```python
from build123d import *

# Parameters (mm, degrees)
F1_DEPTH      = 54.102
F1_DEPTH_BACK = 31.75
F3_DEPTH      = 66.802
F4_R          = 6.35
F6_D          = 25.4
F8_D          = 12.7


with BuildPart() as f1:
    # F0 (on Right) → F1 (new body, two sides)
    with BuildSketch(Plane.YZ) as f1_sk:
        with BuildLine():
            Line((-209.55, 0), (0, 0))
            Line((0, 0), (0, 66.802))
            Line((0, 66.802), (-12.7, 66.802))
            Line((-12.7, 66.802), (-12.7, 16.002))
            Line((-12.7, 16.002), (-69.85, 16.002))
            Line((-69.85, 16.002), (-69.85, 60.452))
            Line((-69.85, 60.452), (-82.55, 60.452))
            Line((-82.55, 60.452), (-82.55, 24.892))
            ThreePointArc((-82.55, 24.892), (-85.153821, 18.605821), (-91.44, 16.002))
            Line((-91.44, 16.002), (-209.55, 16.002))
            Line((-209.55, 16.002), (-209.55, 0))
        make_face()
    extrude(amount=F1_DEPTH)
    extrude(f1_sk.sketch, amount=-F1_DEPTH_BACK)

    # F2 (on Top) → F3 (cut)
    with BuildSketch(Plane.XY):
        with BuildLine():
            Line((31.75, -209.55), (54.102, -209.55))
            Line((54.102, -209.55), (54.102, -12.7))
            Line((54.102, -12.7), (44.45, -12.7))
            ThreePointArc((44.45, -12.7), (35.469744, -16.419744), (31.75, -25.4))
            Line((31.75, -25.4), (31.75, -209.55))
        make_face()
    extrude(amount=F3_DEPTH, mode=Mode.SUBTRACT)

    # F4
    f4_edges = [f1.edges().sort_by_distance(p)[0] for p in [
        (54.102, -6.35, 0),
        (54.102, -6.35, 66.802),
    ]]
    fillet(f4_edges, radius=F4_R)

    # F6 (through all)
    with Locations(Plane.XY.offset(16.002)):
        with Locations((0, -133.35), (0, -184.15)):
            Hole(F6_D / 2)

    # F8 (through all)
    with Locations(Plane.XZ.offset(82.55)):
        with Locations((0, 40.132)):
            Hole(F8_D / 2)


solid = f1.part
```
The model under review builds one solid part; all positions refer to its coordinate system, in mm. A direction names the side the tool comes from. Round coordinates to 2 decimals unless told otherwise and drop trailing zeros. Loops run counter-clockwise (first coordinate to the right, second up) from the corner with the lowest first, then second, coordinate; pieces in that order, holes last.
Item 1: Take a section at C-C (z = 11). Write out the cut boundary in (x, y).
Determined:
outline: (-31.75, -209.55) - (31.75, -209.55) - (31.75, -25.4) arc R12.7 cw to (44.45, -12.7) - (54.1, -12.7) - (54.1, 0) - (-31.75, 0) - close; hole circle Ø25.4 at (0, -184.15); hole circle Ø25.4 at (0, -133.35)
Item 2: Take a section at A-A (x = 0). Write out the cut boundary in (y, z), then the cut area to 3 significant figures.
Determined:
outline: (-209.55, 0) - (-196.85, 0) - (-196.85, 16) - (-209.55, 16) - close; (-171.45, 0) - (-146.05, 0) - (-146.05, 16) - (-171.45, 16) - close; (-120.65, 0) - (0, 0) - (0, 33.78) - (-12.7, 33.78) - (-12.7, 16) - (-69.85, 16) - (-69.85, 33.78) - (-82.55, 33.78) - (-82.55, 24.89) arc R8.89 cw to (-91.44, 16) - (-120.65, 16) - close; (-82.55, 46.48) - (-69.85, 46.48) - (-69.85, 60.45) - (-82.55, 60.45) - close; (-12.7, 46.48) - (0, 46.48) - (0, 66.8) - (-12.7, 66.8) - close
area: 3,440 mm2
Item 3: Clearance check with flat-ended pins moving along their axes: pin 1 Ø10 at (x, y) = (-13, -75.5) entering from +Z; pin 2 Ø4 at (x, z) = (22.5, 19.5) entering from -Y; pin 3 Ø20 at (x, z) = (-1, 42.5) entering from -Y. State where each tip first meets the part, or that it passes through.
Determined:
pin 1: stops at z = 60.45
pin 2: stops at y = -86.5
pin 3: stops at y = -82.55
Item 4: For faces 4 (the face through (0, -69.85, 33)), 5 (the face through (52.192, -6.439, 64.991)), 6 (the face through (31.75, -110, 10)), 7 (the face through (0, -150, 16.002)), 8 (the face through (54.102, -6, 34)), list the 3-axis set-ups (+Z, -Z, +X, -X, +Y, -Y) from which the entire face can be reached by the end or side of a thin tool; tool diameter is ignored.
Determined:
face 4: +Z, +X, -X
face 5: +Z, +X, +Y, -Y
face 6: +Z, -Z, +X, -Y
face 7: +Z, +X, -X, -Y
face 8: +Z, -Z, +X, +Y, -Y
Item 5: Take a section at B-B (y = -133.35). Write out the cut boundary in (x, z), then the cut area to 3 significant figures.
Determined:
outline: (-31.75, 0) - (-12.7, 0) - (-12.7, 16) - (-31.75, 16) - close; (12.7, 0) - (31.75, 0) - (31.75, 16) - (12.7, 16) - close
area: 610 mm2
Item 6: Mouldability with a two-part tool opening along Z and no side actions: class faces 1 (the face through (0, -76, 60.452)), 2 (the face through (0.827, -6.261, 46.428)), 3 (the face through (35.57, -16.32, 7.89)) as released by +Z, released by -Z, zero draft, split by the parting line, or undercut.
Determined:
face 1: released by +Z
face 2: undercut
face 3: zero draft
Item 7: Take a section at D-D (x = 24.5). Write out the cut boundary in (y, z), then the cut area to 3 significant figures.
Determined:
outline: (-209.55, 0) - (0, 0) - (0, 66.8) - (-12.7, 66.8) - (-12.7, 16) - (-69.85, 16) - (-69.85, 60.45) - (-82.55, 60.45) - (-82.55, 24.89) arc R8.89 cw to (-91.44, 16) - (-209.55, 16) - close
area: 4,580 mm2
Item 8: For line 1 (Z direction, x = 0, y = -78); line 2 (Y direction, x = -19, z = 34); line 3 (Z direction, x = 0, y = -9), list the stretches that pass through material, from the lowest coordinate up.
Determined:
line 1: z = 0 to 33.78, 46.48 to 60.45
line 2: y = -82.55 to -69.85, -12.7 to 0
line 3: z = 0 to 33.78, 46.48 to 66.8
